Geometry: see drawing. Coordinates: mm, zero at the bounding-box minimum. A direction names the side the tool comes from. Round coordinates to 2 decimals unless told otherwise and drop trailing zeros. Write each loop counter-clockwise with the first axis right and the second up, starting at its lowest first coordinate (ties: lowest second). Pieces come first, ordered by that corner, then holes. Notation, with made-up numbers: M 52,-20 L 74,-20 A15 cw 74,9 Z; hole C 61.5,13.5 d7. An arc over 180 degrees is marked long. Use a Markdown table: item, result.
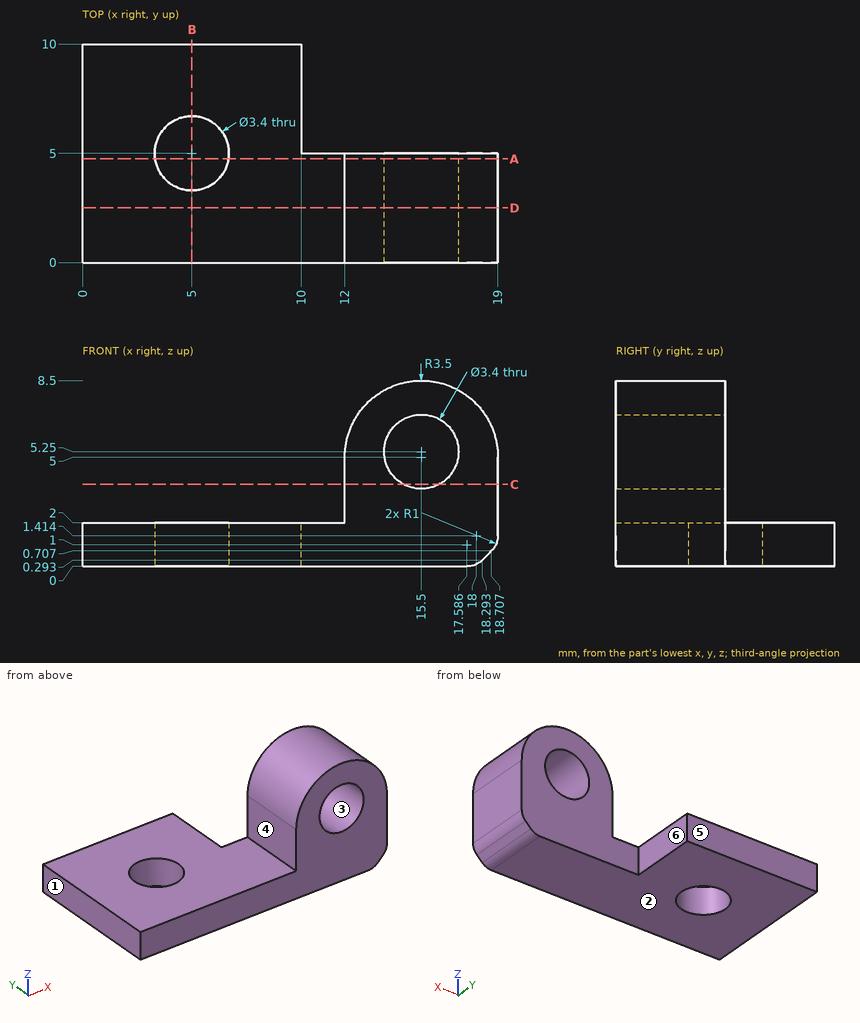
Q1. Mould query, pull axis Z, two halves, no side actions, for the marked faces 1, 2 and 3. Classes: +Z half, -Z half, draft (parallel to the pull), parting line (faces both ways), or undercut.
Results are:
| item | result |
|---|---|
| face 1 | draft |
| face 2 | -Z half |
| face 3 | undercut |
Q2. Section C-C on z = 3.75. Return loops of the section in (x, y), plus the area to 3 significant figures.
Results are:
| item | result |
|---|---|
| outline | M 12,0 L 14.7,0 L 14.7,5 L 12,5 Z; M 16.3,0 L 19,0 L 19,5 L 16.3,5 Z |
| area | 27.0 mm^2 |
Q3. First-contact query: pin 1 Ø4.5 at (x, z) = (15.5, 5.25) entering from +Y; pin 2 Ø0.6 at (y, z) = (6.5, 1) entering from +X; pin 3 Ø0.9 at (y, z) = (2, 3.5) entering from -X. Flat tips, straight axial feed; report the tip coordinate or a pass-through.
Results are:
| item | result |
|---|---|
| pin 1 | y = 5 |
| pin 2 | x = 10 |
| pin 3 | x = 12 |
Q4. Line query: L1, parallel to Z at x = 15.5, y = 1.9; L2, parallel to Y at x = 15.25, z = 8.25; L3, parallel to Z at x = 11.75, y = 3. Output: solid intervals per line, ascending.
Results are:
| item | result |
|---|---|
| L1 | 0 to 3.55, 6.95 to 8.5 |
| L2 | 0 to 5 |
| L3 | 0 to 2 |
Q5. Section D-D on y = 2.5. Return loops of the section in (x, z), plus the area to 3 significant figures.
Results are:
| item | result |
|---|---|
| outline | M 0,0 L 17.59,0 A1 ccw 18.29,0.29 L 18.71,0.71 A1 ccw 19,1.41 L 19,5 A3.5 ccw 12,5 L 12,2 L 0,2 Z; hole C 15.5,5.25 d3.4 |
| area | 68.6 mm^2 |
Q6. Section A-A on y = 4.75. Return loops of the section in (x, z).
Results are:
| item | result |
|---|---|
| outline | M 0,0 L 3.32,0 L 3.32,2 L 0,2 Z; M 6.68,0 L 17.59,0 A1 ccw 18.29,0.29 L 18.71,0.71 A1 ccw 19,1.41 L 19,5 A3.5 ccw 12,5 L 12,2 L 6.68,2 Z; hole C 15.5,5.25 d3.4 |
Q7. Reachability of the marked faces 4, 5 and 6 from +Z, -Z, +X, -X, +Y, -Y: full face, straight path, thin tool, end or side. Return the list, or none.
Results are:
| item | result |
|---|---|
| face 4 | +Z, -X, +Y, -Y |
| face 5 | +Z, -Z, +X, -X, +Y |
| face 6 | +Z, -Z, +X, +Y |
Q8. Section B-B on x = 5. Return loops of the section in (y, z), plus the area to 3 significant figures.
Results are:
| item | result |
|---|---|
| outline | M 0,0 L 3.3,0 L 3.3,2 L 0,2 Z; M 6.7,0 L 10,0 L 10,2 L 6.7,2 Z |
| area | 13.2 mm^2 |
